Part model, mm, in its own coordinate system. Face numbers are marked on the shaded views. A direction names the side the tool comes from. Round coordinates to 2 decimals unless told otherwise and drop trailing zeros. Write each loop counter-clockwise with the first axis right and the second up, starting at its lowest first coordinate (ties: lowest second). Pieces come first, ordered by that corner, then holes. Notation, with made-up numbers: (-19.75, 80) -> (16.25, 80) arc R14 cw to (16.25, 102) -> close; hole circle Ø8 at (-27.5, -34). An arc over 180 degrees is marked (long way). Return JSON: item names as keys, results as strings. Group by question number.
(1) Tool access for the marked faces 5 and 6: list every direction of +Z, -Z, +X, -X, +Y, -Y with a clear straight run to the whole face (end or side of a thin tool).
(2) Drill centre lines: L1, parallel to Y at x = -0.5, z = 70; L2, parallel to Y at x = 1.5, z = 18; L3, parallel to X at y = 0, z = 52. Where is each one in solid material? Low to high. Write a range as from..to.
(3) Drop flat-ended pins along their axis: pin 1 Ø10 at (x, z) = (-3, 20.5) entering from -Y; pin 2 Ø12 at (y, z) = (28, 57) entering from -X; pin 3 Ø16 at (x, y) = (0, 0) entering from -Z; pin 4 Ø1 at (x, z) = (17, 63.5) entering from +Y. Give the stop position or say it passes through.
(4) Saw through at A-A (z = 16). List the corners of the cut face in (x, y).
(5) Mould opens along X. For the marked faces 1, 2, 3 and 4 say: +X half, -X half, draft (parallel to the pull), parting line (faces both ways), or undercut.
from build123d import *

# Parameters (mm, degrees)
F1_DEPTH       = 73.5
F3_D           = 20
F3_CBORE_D     = 20
F3_CBORE_DEPTH = 20
F4_R           = 5


# Not quite as in the source:
# - two fillets or chamfers of one size are made in one step


with BuildPart() as f1:
    # F0 (on Top) → F1 (new body)
    with BuildSketch(Plane.XY):
        Polygon((-1.1557375875, 37.9352838977), (-30.379589847, 22.7486706094), (-36.726991321, -9.568155636), (-15.4182192362, -34.6799655328), (17.5007864078, -33.6770540409), (37.2413429358, -7.3146339696), (28.9384086481, 24.5558546722), align=None)
    extrude(amount=F1_DEPTH)

    # F3 (through all)
    with Locations(Plane.XY.offset(73.5)):
        with Locations((0, 0)):
            CounterBoreHole(F3_D / 2, F3_CBORE_D / 2, F3_CBORE_DEPTH)

    # F4
    f4_edges = [f1.edges().sort_by_distance(p)[0] for p in [
        (-26.072605, -22.124061, 0),
        (-33.553291, 6.590257, 0),
        (-36.726991, -9.568156, 36.75),
        (-15.418219, -34.679966, 36.75),
        (-33.553291, 6.590257, 73.5),
        (-26.072605, -22.124061, 73.5),
        (-15.767664, 30.341977, 73.5),
        (-30.37959, 22.748671, 36.75),
        (-1.155738, 37.935284, 36.75),
        (28.938409, 24.555855, 36.75),
        (13.891336, 31.245569, 73.5),
        (33.089876, 8.62061, 73.5),
        (13.891336, 31.245569, 0),
        (33.089876, 8.62061, 0),
        (1.041284, -34.17851, 0),
        (27.371065, -20.495844, 0),
        (17.500786, -33.677054, 36.75),
        (37.241343, -7.314634, 36.75),
        (1.041284, -34.17851, 73.5),
        (27.371065, -20.495844, 73.5),
        (-15.767664, 30.341977, 0),
        (-10, 0, 0),
        (-10, 0, 73.5),
    ]]
    fillet(f4_edges, radius=F4_R)


solid = f1.part
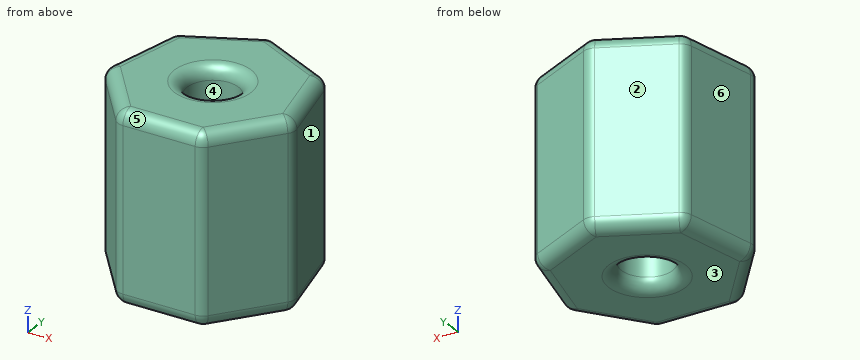
Computed values:
{
 "1": {"face 5": "+Z, +X, -Y", "face 6": "+Z, -Z, -X, +Y"},
 "2": {"L1": "-34..-10.22, 10.22..37.13", "L2": "-34.16..-9.89, 9.89..36.75", "L3": "-34.85..-10, 10..35.34"},
 "3": {"pin 1": "y = -34.45", "pin 2": "x = -30.22", "pin 3": "through", "pin 4": "y = 30.09"},
 "4": {"outline": "(-36.26, -7.21) arc R5 ccw to (-35.17, -11.4) -> (-16.98, -32.84) arc R5 ccw to (-13.01, -34.61) -> (15.09, -33.75) arc R5 ccw to (18.94, -31.75) -> (35.8, -9.24) arc R5 ccw to (36.63, -4.98) -> (29.55, 22.23) arc R5 ccw to (26.74, 25.53) -> (1.04, 36.96) arc R5 ccw to (-3.29, 36.82) -> (-28.24, 23.86) arc R5 ccw to (-30.84, 20.39) -> close; hole circle Ø20 at (0, 0)"},
 "5": {"face 1": "+X half", "face 2": "-X half", "face 3": "draft", "face 4": "undercut"}
}
